Verification items for the finished model (mm, model axes). A direction names the side the tool comes from. Coordinates: 2 decimals unless noted, no trailing zeros. Order: outer loops, then holes, each group sorted by start corner. A loop starts at its lowest first (then second) coordinate and runs counter-clockwise, first axis right, second up. Notation, with made-up numbers: (5, 25) -> (46, 25) arc R29 ccw to (46, 56) -> close; hole circle Ø11 at (79.5, -35.75). An arc over 180 degrees is marked (long way). Use CSV: the item, a comma, the result in double quotes. Start each with the question number.
1) Tool access check on faces 1 (the flat face through (31.855, -0.2, -9.5)), 2 (the flat face through (313, 31, 71)), 3 (the flat face through (37, -14.5, 156)), 4 (the flat face through (37, -14.5, -11)). Record the directions out of +Z, -Z, +X, -X, +Y, -Y that give a thin tool (end or side, any length) a straight path to the whole face; none if there is none.
2) Sectioned sample at D-D on x = 340. Record the boundary of the cut face in (y, z).
3) Go/stop test with flat-tipped pins: pin 1 (3 mm diameter, centred on y = -31.5, z = 167.5, fed in from +X) (3 decimals); pin 2 (10 mm diameter, centred on x = 326.5, y = 21.5, fed in from -Z); pin 3 (4 mm diameter, centred on x = 55, z = 6, fed in from -Y). Record where each tip stops, or that it passes through.
4) Release check for a two-part mould opening along Y. For faces 5 (the flat face through (196, 33, 82)), 6 (the flat face through (31.855, 31.3, 72.9)), 7 (the cylindrical face through (394.16, -1.72, -1.97)) record: released by +Y, released by -Y, zero draft, split by the parting line, or undercut.
5) Sectioned sample at A-A on z = 117. Record the boundary of the cut face in (x, y) (1 decimal).
6) Scan lines: line 1 along Z through (x, y) = (351.5, 0); line 2 along Z through (x, y) = (130, -11.5); line 3 along Y through (x, z) = (260, 147). Record each from-to range of solid material in increasing order.
7) Sectioned sample at C-C on x = 390. Record the boundary of the cut face in (y, z).
8) Sectioned sample at B-B on y = -37. Record the boundary of the cut face in (x, z) (3 decimals).
Autodesk Inventor part; units mm, degrees
ref_plane "Płaszczyzna konstrukcyjna1" through (117.8756, 33, 145) normal (0, 0, 1) x (-1, 0, 0)
ref_plane "Płaszczyzna konstrukcyjna4" through (117.8756, 33, 72.5) normal (0, 0, -1) x (-1, 0, 0)
ref_plane "Płaszczyzna konstrukcyjna6" through (0, 0, 72.5) normal (0, 0, 1) x (1, 0, 0)
sketch "Szkic1" plane through (0, 0, 0) normal (0, 0, 1) x (1, 0, 0)
  arc A0 (0, 35) -> (0, -35) centre (0, 0) ccw construction
  line L0 (0, 35) -> (390, 35) construction
  line L1 (0, -35) -> (390, -35) construction
  arc A1 (390, -35) -> (390, 35) centre (390, 0) ccw construction
  circle A2 centre (0, 0) radius 4.5
  circle A3 centre (390, 0) radius 4.5
  line L2 (130, 35) -> (130, 10) construction
  line L3 (260, 35) -> (260, 10) construction
  circle A4 centre (130, 10) radius 25 construction
  circle A5 centre (260, 10) radius 25 construction
  circle A6 centre (130, 10) radius 4.5
  circle A7 centre (260, 10) radius 4.5
  circle A8 centre (0, 0) radius 35 construction
  circle A9 centre (390, 0) radius 35 construction
  line L4 (117.8756, 33) -> (31.8551, 33)
  line L5 (375.6125, 33) -> (272.1244, 33)
  line L6 (247.8756, 33) -> (142.1244, 33)
  line L7 (31.8551, 31) -> (114.6703, 31)
  line L8 (145.3297, 31) -> (244.6703, 31)
  line L9 (275.3297, 31) -> (371.697, 31)
  arc A10 (375.6125, 33) -> (371.697, 31) centre (390, 0) ccw
  arc A11 (117.8756, 33) -> (114.6703, 31) centre (130, 10) ccw
  arc A12 (145.3297, 31) -> (142.1244, 33) centre (130, 10) ccw
  arc A13 (247.8756, 33) -> (244.6703, 31) centre (260, 10) ccw
  arc A14 (275.3297, 31) -> (272.1244, 33) centre (260, 10) ccw
  line L10 (31.8551, 14.5) -> (31.8551, 35) construction
  line L11 (31.8551, 33) -> (31.8551, 31)
  line L12 (260, 10) -> (260, 0)
  line L13 (130, 10) -> (130, 0)
  point P0 (423.5971, -9.8098)
  dimension "d94" = 50
  dimension "d0" = 70
  dimension "d1" = 390
  dimension "d2" = 390
  dimension "d3" = 70
  dimension "d4" = 9
  dimension "d5" = 9
  dimension "d10" = 25
  dimension "d11" = 25
  dimension "d12" = 9
  dimension "d13" = 9
  dimension "d14" = 130
  dimension "d15" = 260
  dimension "d24" = 2
  dimension "d25" = 2
  dimension "d26" = 2
  dimension "d27" = 1
  dimension "d95" = 2
extrude "Wyciągnięcie proste1" add sketch "Szkic1" along normal blind 145 contours A11 L7 L11 L4 | A10 L9 A14 L5 | A13 L8 A12 L6
ref_plane "Płaszczyzna konstrukcyjna1" through (117.8756, 33, 145) normal (0, 0, 1) x (-1, 0, 0)
sketch "Szkic3" plane through (117.8756, 33, 145) normal (0, 0, 1) x (-1, 0, 0)
  circle A0 centre (117.8756, 33) radius 4.5
  arc A1 (133.7659, 28.5) -> (133.7659, 37.5) centre (133.7659, 33) ccw
  arc A2 (98.6659, 37.5) -> (98.6659, 28.5) centre (98.6659, 33) ccw
  line L0 (133.7659, 28.5) -> (98.6659, 28.5)
  line L1 (98.6659, 37.5) -> (133.7659, 37.5)
  line L2 (98.6659, 18.5) -> (133.7659, 18.5)
  arc A3 (133.7659, 18.5) -> (133.7659, 47.5) centre (133.7659, 33) ccw
  line L3 (133.7659, 47.5) -> (98.6659, 47.5)
  line L4 (86.0205, 18.5) -> (86.0205, -2) construction
  line L5 (98.6659, 18.5) -> (86.0205, 18.5)
  line L6 (98.6659, 47.5) -> (86.0205, 47.5)
  line L7 (86.0205, 0) -> (86.0205, 2)
  line L8 (86.0205, 18.5) -> (86.0205, 0)
  line L9 (98.6659, 47.5) -> (98.6659, 81.8113)
  line L10 (98.6659, 81.8113) -> (-234.1244, 81.8113)
  line L11 (-157.4541, 2) -> (-253.8214, 2)
  line L12 (86.0205, 0) -> (86.0205, 2)
  line L13 (-257.7369, 0) -> (-154.2487, 0)
  line L14 (86.0205, 0) -> (-238.0399, 0)
  circle A4 centre (-272.1244, 33) radius 35 construction
  line L15 (-234.1244, 2) -> (-234.1244, 18.5)
  line L16 (-234.1244, 2) -> (-238.0399, 0)
  line L17 (-246.7694, 47.5) -> (-246.7694, 81.8113)
  line L18 (-246.7694, 81.8113) -> (-234.1244, 81.8113)
  line L19 (-303.9795, 47.5) -> (-409.6259, 47.5) construction
  line L20 (-234.1244, 47.5) -> (-246.7694, 47.5)
  line L21 (-234.1244, 18.5) -> (-281.8694, 18.5)
  line L22 (-246.7694, 47.5) -> (-281.8694, 47.5)
  arc A5 (-281.8694, 47.5) -> (-281.8694, 18.5) centre (-281.8694, 33) ccw
  point P0 (-238.0399, 0)
  dimension "d33" = 9
  dimension "d34" = 9
  dimension "d35" = 10
  dimension "d36" = 47.7454
  dimension "d37" = 12.6455
  dimension "d38" = 12.6455
  dimension "d39" = 12.6455
  dimension "d40" = 0
  dimension "d64" = 47.745
  dimension "d93" = 16.5
extrude "Wyciągnięcie proste2" add sketch "Szkic3" along normal blind 4
ref_plane "Płaszczyzna konstrukcyjna4" through (117.8756, 33, 72.5) normal (0, 0, -1) x (-1, 0, 0)
mirror "Odbij2" about plane through (117.8756, 33, 72.5) normal (0, 0, -1) of "Wyciągnięcie proste2"
extrude "Wyciągnięcie proste4" cut sketch "Szkic1" along normal mid plane 10000 contours A6 | A7
sketch "Szkic8" plane through (0, 0, 145) normal (0, 0, 1) x (1, 0, 0)
  line L0 (352, 31) -> (371.697, 31)
  line L1 (352, 31) -> (355.9155, 33)
  line L2 (352, 31) -> (355.9155, 33)
  line L3 (375.6125, 33) -> (355.9155, 33)
  line L4 (355.9155, 33) -> (375.6125, 33)
  arc A0 (375.6125, 33) -> (371.697, 31) centre (390, 0) ccw
  line L5 (375.6125, 33) -> (371.697, 31)
  line L6 (352, 14.5) -> (352, 31)
  line L7 (371.697, 31) -> (352, 31)
  point P0 (0, 0)
  point P1 (352, -48.8113)
ref_plane "Płaszczyzna konstrukcyjna6" through (0, 0, 72.5) normal (0, 0, 1) x (1, 0, 0)
extrude "Wyciągnięcie proste5" cut sketch "Szkic8" along normal mid plane 1000 contours L1 L3 A0 L0
ref_plane "Płaszczyzna konstrukcyjna9" through (117.8756, 33, 149) normal (0, 0, 1) x (1, 0, 0)
sketch "Szkic12" plane through (117.8756, 33, 149) normal (0, 0, 1) x (1, 0, 0)
  line L0 (281.8694, -18.5) -> (234.1244, -18.5)
  arc A0 (281.8694, -47.5) -> (281.8694, -18.5) centre (281.8694, -33) ccw
  line L1 (246.7694, -47.5) -> (281.8694, -47.5)
  line L2 (246.7694, -81.8113) -> (246.7694, -47.5)
  line L3 (234.1244, -2) -> (234.1244, -81.8113)
  line L4 (-98.6659, -81.8113) -> (246.7694, -81.8113)
  point P0 (-117.8756, -33)
extrude "Wyciągnięcie proste7" cut sketch "Szkic12" against normal blind 17
extrude "Wyciągnięcie proste8" cut sketch "Szkic1" against normal blind 17 contours A3
ref_plane "Płaszczyzna konstrukcyjna10" through (117.8756, 33, 149) normal (0, 0, 1) x (1, 0, 0)
sketch "Szkic13" plane through (117.8756, 33, 149) normal (0, 0, 1) x (1, 0, 0)
  line L0 (234.1244, -81.8113) -> (234.1244, -2)
  line L1 (232.1244, -81.8113) -> (232.1244, -2)
  line L2 (234.1244, -2) -> (238.0399, 0)
  line L3 (238.0399, 0) -> (236.0399, 0)
  line L4 (238.0399, 0) -> (-86.0205, 0)
  line L5 (236.0399, 0) -> (232.1244, -2)
  line L6 (238.0399, 0) -> (234.1244, -2)
  line L7 (234.1244, -81.8113) -> (232.1244, -81.8113)
  line L8 (-98.6659, -81.8113) -> (246.7694, -81.8113)
  point P0 (-117.8756, -33)
  dimension "d70" = 2
  dimension "d71" = 2
extrude "Wyciągnięcie proste9" add sketch "Szkic13" along normal blind 17
ref_plane "Płaszczyzna konstrukcyjna11" through (117.8756, 33, 166) normal (0, 0, 1) x (1, 0, 0)
sketch "Szkic14" plane through (117.8756, 33, 166) normal (0, 0, 1) x (1, 0, 0)
  line L0 (232.1244, -81.8113) -> (234.1244, -81.8113)
  line L1 (-98.6659, -81.8113) -> (246.7694, -81.8113)
  line L2 (232.1244, -81.8113) -> (246.7694, -81.8113)
  line L3 (246.7694, -81.8113) -> (246.7694, -47.5)
  line L4 (246.7694, -81.8113) -> (246.7694, -47.5)
  line L5 (246.7694, -47.5) -> (281.8694, -47.5)
  line L6 (246.7694, -47.5) -> (281.8694, -47.5)
  line L7 (281.8694, -18.5) -> (234.1244, -18.5)
  line L8 (234.1244, -81.8113) -> (234.1244, -2)
  arc A0 (281.8694, -47.5) -> (281.8694, -18.5) centre (281.8694, -33) ccw
  circle A1 centre (272.1244, -33) radius 4.5
  line L9 (232.1244, -2) -> (232.1244, -81.8113)
  line L10 (236.0399, 0) -> (232.1244, -2)
  line L11 (238.0399, 0) -> (236.0399, 0)
  line L12 (234.1244, -2) -> (238.0399, 0)
  point P0 (-117.8756, -33)
extrude "Wyciągnięcie proste10" add sketch "Szkic14" along normal blind 4
ref_plane "Płaszczyzna konstrukcyjna12" through (364.645, -48.8113, -4) normal (0, 0, -1) x (-1, 0, 0)
sketch "Szkic15" plane through (364.645, -48.8113, -4) normal (0, 0, -1) x (-1, 0, 0)
  line L0 (332.7899, 63.3113) -> (322.7899, 63.3113)
  line L1 (322.7899, 63.3113) -> (322.7899, 34.3113)
  line L2 (322.7899, 34.3113) -> (332.7899, 34.3113)
  line L3 (332.7899, 34.3113) -> (332.7899, 63.3113)
  point P0 (364.645, 48.8113)
  dimension "d78" = 10
extrude "Wyciągnięcie proste11" add sketch "Szkic15" along normal blind 14.44
ref_plane "Płaszczyzna konstrukcyjna13" through (117.8756, 33, 149) normal (0, 0, 1) x (1, 0, 0)
sketch "Szkic16" plane through (117.8756, 33, 149) normal (0, 0, 1) x (1, 0, 0)
  line L0 (-86.0205, -18.5) -> (-133.7659, -18.5)
  line L1 (-86.0205, -47.5) -> (-76.0205, -47.5)
  line L2 (-86.0205, -18.5) -> (-76.0205, -18.5)
  line L3 (-76.0205, -18.5) -> (-76.0205, -47.5)
  line L4 (-76.0205, -47.5) -> (-86.0205, -47.5)
  line L5 (-86.0205, -47.5) -> (-86.0205, -18.5)
  point P0 (-117.8756, -33)
  point P1 (-86.0205, -47.5)
  dimension "d82" = 10
extrude "Wyciągnięcie proste12" add sketch "Szkic16" along normal blind 14.44
ref_plane "Płaszczyzna konstrukcyjna14" through (31.8551, -14.5, -4) normal (-1, 0, 0) x (0, 0, 1)
sketch "Szkic17" plane through (31.8551, -14.5, -4) normal (-1, 0, 0) x (0, 0, 1)
  line L0 (4, 0) -> (4, 29)
  line L1 (4, 19) -> (-14.44, 19)
  line L2 (-14.44, 29) -> (-14.44, 0)
  line L3 (4, 10) -> (0, 10)
  line L4 (4, 10) -> (-12.44, 10)
  line L5 (4, 18.5) -> (-12.44, 18.5)
  line L6 (-12.44, 18.5) -> (-4.44, 18.5)
  line L7 (-4.44, 18.5) -> (-4.44, 10.5)
  line L8 (-4.44, 10.5) -> (-12.44, 10.5)
  line L9 (-12.44, 10.5) -> (-12.44, 18.5)
  circle A0 centre (-8.44, 14.5) radius 2.5
  point P0 (4, 14.5)
  dimension "d86" = 9
  dimension "d87" = 0.5
  dimension "d88" = 8
  dimension "d89" = 8
  dimension "d90" = 5
extrude "Wyciągnięcie proste13" cut sketch "Szkic17" against normal through all contours A0
mirror "Odbij3" about plane through (117.8756, 33, 72.5) normal (0, 0, -1) of "Wyciągnięcie proste13"
sketch "Szkic20" plane through (117.8756, 33, 72.5) normal (0, 0, 1) x (-1, 0, 0)
  point P0 (117.8756, -33)
ref_plane "Płaszczyzna konstrukcyjna5" through (117.8756, 33, 72.5) normal (0, 0, -1) x (-1, 0, 0)
properties part number "Podstawa"
Answers follow:
1,face 1,"-Z, -X, +Y, -Y"
1,face 2,"+X, -X, -Y"
1,face 3,"+Z, -X, -Y"
1,face 4,"-Z, +X, -X, -Y"
2,outline,"(-48.81, -4) -> (33, -4) -> (33, 149) -> (-48.81, 149) -> (-48.81, 145) -> (31, 145) -> (31, 0) -> (-48.81, 0) -> close"
3,pin 1,"stops at x = 364.645"
3,pin 2,"stops at z = -4"
3,pin 3,"stops at y = 31"
4,face 5,"released by +Y"
4,face 6,"zero draft"
4,face 7,"undercut"
5,outline,"(31.9, 31) -> (114.7, 31) arc R26 cw to (117.9, 33) -> (31.9, 33) -> close; (142.1, 33) arc R26 cw to (145.3, 31) -> (244.7, 31) arc R26 cw to (247.9, 33) -> close; (272.1, 33) arc R26 cw to (275.3, 31) -> (352, 31) -> (355.9, 33) -> close"
6,line 1,"z = -4 to 0, 145 to 154.94, 159.94 to 170"
6,line 2,"z = -4 to 0, 145 to 149"
6,line 3,"y = -48.81 to 5.5, 14.5 to 33"
7,outline,"(-14.5, -4) -> (-4.5, -4) -> (-4.5, 0) -> (-14.5, 0) -> close; (-14.5, 166) -> (-4.5, 166) -> (-4.5, 170) -> (-14.5, 170) -> close; (4.5, -4) -> (14.5, -4) -> (14.5, 0) -> (4.5, 0) -> close; (4.5, 166) -> (14.5, 166) -> (14.5, 170) -> (4.5, 170) -> close"
8,outline,"(19.21, -4) -> (364.645, -4) -> (364.645, 0) -> (19.21, 0) -> close; (19.21, 145) -> (352, 145) -> (352, 166) -> (364.645, 166) -> (364.645, 170) -> (350, 170) -> (350, 149) -> (19.21, 149) -> close"
